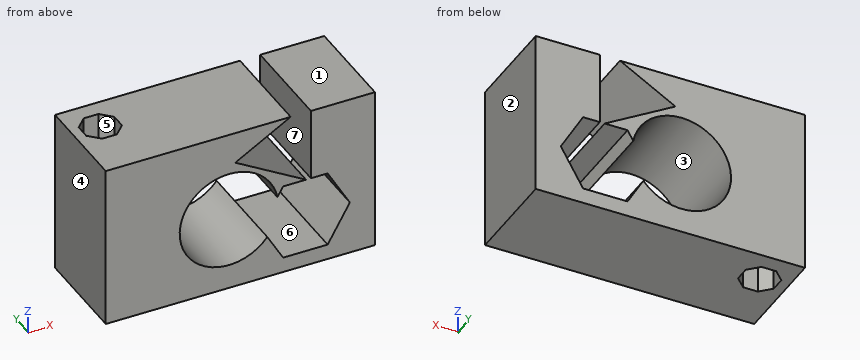
from build123d import *

# Parameters (mm, degrees)
F0_W     = 69.364339
F0_H     = 42.640485
F1_DEPTH = 25.4
F2_R     = 12.7
F3_DEPTH = 25.401
F4_DEPTH = 19.05
F6_DEPTH = 25.4
F8_DEPTH = 42.641485


with BuildPart() as f1:
    # F0 (on Front) → F1 (new body)
    with BuildSketch(Plane.XZ):
        with Locations((34.68217, 21.320242)):
            Rectangle(F0_W, F0_H)
    extrude(amount=F1_DEPTH)

    # F2 (on face) → F3 (cut, through all)
    with BuildSketch(Plane.XZ.offset(25.4)):
        with Locations((31.75, 19.05)):
            Circle(F2_R)
        Polygon((52.866902, 23.142773), (52.866902, 45.649943), (33.375122, 34.396358), align=None)
    extrude(amount=-F3_DEPTH, mode=Mode.SUBTRACT)

    # F2 (on face) → F4 (cut)
    with BuildSketch(Plane.XZ.offset(25.4)):
        with Locations((31.75, 19.05)):
            Circle(F2_R)
        Polygon((52.866902, 23.142773), (52.866902, 45.649943), (33.375122, 34.396358), align=None)
    extrude(amount=-F4_DEPTH, mode=Mode.SUBTRACT)

    # F5 (on face) → F6 (cut)
    with BuildSketch(Plane.XZ.offset(25.4)):
        Polygon((45.705261, 4.008082), (57.173451, 4.008082), (62.907545, 13.939825), (57.173451, 23.871568), (45.705261, 23.871568), (39.971167, 13.939825), align=None)
    extrude(amount=-F6_DEPTH, mode=Mode.SUBTRACT)

    # F7 (on face) → F8 (cut, through all)
    with BuildSketch(Plane.XY.offset(42.640485)):
        Polygon((5.218119, -13.429749), (9.02866, -13.429749), (11.72312, -10.735289), (11.72312, -6.924748), (9.02866, -4.230288), (5.218119, -4.230288), (2.523659, -6.924748), (2.523659, -10.735289), align=None)
    extrude(amount=-F8_DEPTH, mode=Mode.SUBTRACT)


solid = f1.part
Verification items for the finished model (mm, model axes). Face numbers are marked on the shaded views. A direction names the side the tool comes from. Round coordinates to 2 decimals unless told otherwise and drop trailing zeros. Order: outer loops, then holes, each group sorted by start corner. A loop starts at its lowest first (then second) coordinate and runs counter-clockwise, first axis right, second up. Notation, with made-up numbers: (-25.75, -14.5) -> (19.25, -14.5) arc R21 cw to (19.25, 11.5) -> close; hole circle Ø11 at (33, 63). An arc over 180 degrees is marked (long way). Put each result on its own line as item: value.
1) Section check D-D (x = 40). Record the cut outline in (y, z).
Final values:
outline: (-25.4, 0) -> (0, 0) -> (0, 9.39) -> (-25.4, 9.39) -> close; (-25.4, 28.71) -> (0, 28.71) -> (0, 30.57) -> (-25.4, 30.57) -> close; (-25.4, 38.22) -> (0, 38.22) -> (0, 42.64) -> (-25.4, 42.64) -> close
2) Section check B-B (x = 58). Record the cut outline in (y, z), then the cut area to 3 significant figures.
Final values:
outline: (-25.4, 0) -> (0, 0) -> (0, 5.44) -> (-25.4, 5.44) -> close; (-25.4, 22.44) -> (0, 22.44) -> (0, 42.64) -> (-25.4, 42.64) -> close
area: 651 mm^2
3) Material ranges on line 1 (X direction, y = -9.5, z = 30); line 2 (Z direction, x = 37.5, y = -10.25); line 3 (Y direction, x = 8.5, z = 11), recorded low to high.
Final values:
line 1: x = 0 to 2.52, 11.72 to 25.32, 38.18 to 40.99, 52.87 to 69.36
line 2: z = 0 to 7.73, 30.37 to 32.01, 36.78 to 42.64
line 3: y = -25.4 to -13.43, -4.23 to 0
4) Section check A-A (z = 8). Record the cut outline in (x, y).
Final values:
outline: (0, -25.4) -> (25.49, -25.4) -> (25.49, 0) -> (0, 0) -> close; (38.01, -25.4) -> (43.4, -25.4) -> (43.4, 0) -> (38.01, 0) -> close; (59.48, -25.4) -> (69.36, -25.4) -> (69.36, 0) -> (59.48, 0) -> close; hole (2.52, -10.74) -> (5.22, -13.43) -> (9.03, -13.43) -> (11.72, -10.74) -> (11.72, -6.92) -> (9.03, -4.23) -> (5.22, -4.23) -> (2.52, -6.92) -> close
5) Depth check by flat-ended pin: pin 1 (15 mm diameter, centred on x = 31.75, z = 19.05, fed in from +Y); pin 2 (1.1 mm diameter, centred on x = 7.5, z = 29, fed in from +Y). Enter the tip coordinate at first touch or a pass-through.
Final values:
pin 1: passes through
pin 2: stops at y = 0
6) Section check C-C (z = 33). Record the cut outline in (x, y).
Final values:
outline: (0, -25.4) -> (35.79, -25.4) -> (35.79, 0) -> (0, 0) -> close; (52.87, -25.4) -> (69.36, -25.4) -> (69.36, 0) -> (52.87, 0) -> close; hole (2.52, -10.74) -> (5.22, -13.43) -> (9.03, -13.43) -> (11.72, -10.74) -> (11.72, -6.92) -> (9.03, -4.23) -> (5.22, -4.23) -> (2.52, -6.92) -> close
7) Mould release check, pull along X, two halves, no side actions. Record for the marked faces 1, 2, 3 and 4: +X half, -X half, draft (parallel to the pull), parting line (faces both ways), or undercut.
Final values:
face 1: draft
face 2: +X half
face 3: undercut
face 4: -X half
8) Set-up check for the marked faces 5, 6 and 7: record each of +Z, -Z, +X, -X, +Y, -Y from which the full face is reachable in a straight line by a thin tool's end or side.
Final values:
face 5: +Z, -Z
face 6: +Y, -Y
face 7: +Z, +Y, -Y
